The listing builds one solid part. Answer for the finished solid, in the listing's coordinates (mm). A direction names the side the tool comes from. Coordinates: 2 decimals unless noted, no trailing zeros. Loops run counter-clockwise (first coordinate to the right, second up) from the corner with the lowest first, then second, coordinate; pieces in that order, holes last. Notation, with made-up numbers: M 44,-39 L 83,-39 A19 ccw 83,-26 Z; hole C 56.5,59 d8. An arc over 180 degrees is marked long. Return JSON: item names as keys, results as strings. Group by question number.
1. Section C-C (z = 29) is taken. Write down the section's boundary in (x, y).
2. Section D-D (y = 0) is taken. Write down the section's boundary in (x, z).
3. Given P1, Ø6, axis at x = -2.5, y = 39.5, coming from the +Z side, flat-ended and moving along its own axis, determine where the tip first touches the part or whether it passes through.
4. Section B-B (x = 31) is taken. Write down the section's boundary in (y, z), then the cut area to 3 significant figures.
5. Which of the six approach directions +Z, -Z, +X, -X, +Y, -Y give full straight-line access (tool end or side, diameter ignored) to faces 4 (the face through (-51, 1, 76.2)), 5 (the face through (-50.062, -1, 38)), 6 (the face through (26.223, -39, 63))?
6. Straight lines are drawn through the part: L1, parallel to X at y = 3, z = 32; L2, parallel to Y at x = 40, z = 63.5; L3, parallel to Z at x = -52.5, y = 0. For each, find the intervals that lie inside material, in ascending order. Write a range as from..to.
7. Section A-A (y = 24.5) is taken. Write down the section's boundary in (x, z).
8. The mould has two halves that part along Y. Classify faces 1 (the face through (26.223, 39, 63)), 2 (the face through (52.782, -1.485, 63.907)), 3 (the face through (-1, 41.569, 29)): pulls with the +Y half, pulls with the -Y half, needs draft (parallel to the pull), parting line crosses it, or undercut.
```python
from build123d import *

# Parameters (mm, degrees)
F0_W     = 110.851846
F0_H     = 83.138884
F0_W_2   = 100.124248
F0_H_2   = 71.815304
F1_DEPTH = 76.2
F2_W     = 52.446034
F2_H     = 26.882852
F3_DEPTH = 103.124
F4_R     = 11.409512
F5_DEPTH = 113.538


with BuildPart() as f1:
    # F0 (on Top) → F1 (new body)
    with BuildSketch(Plane.XY):
        Rectangle(F0_W, F0_H)
        Rectangle(F0_W_2, F0_H_2, mode=Mode.SUBTRACT)
    extrude(amount=F1_DEPTH)

    # F2 (on face) → F3 (cut)
    with BuildSketch(Plane.XZ.offset(41.569442)):
        with Locations((0, 62.758574)):
            Rectangle(F2_W, F2_H)
    extrude(amount=-F3_DEPTH, mode=Mode.SUBTRACT)

    # F4 (on face) → F5 (cut)
    with BuildSketch(Plane.YZ.offset(55.425923)):
        with Locations((0, 52.595027)):
            Circle(F4_R)
    extrude(amount=-F5_DEPTH, mode=Mode.SUBTRACT)


solid = f1.part
```
Worked out:
{
 "1": {"outline": "M -55.43,-41.57 L 55.43,-41.57 L 55.43,41.57 L -55.43,41.57 Z; hole M -50.06,-35.91 L 50.06,-35.91 L 50.06,35.91 L -50.06,35.91 Z"},
 "2": {"outline": "M -55.43,0 L -50.06,0 L -50.06,41.19 L -55.43,41.19 Z; M -55.43,64 L -50.06,64 L -50.06,76.2 L -55.43,76.2 Z; M 50.06,0 L 55.43,0 L 55.43,41.19 L 50.06,41.19 Z; M 50.06,64 L 55.43,64 L 55.43,76.2 L 50.06,76.2 Z"},
 "3": {"P1": "z = 49.32"},
 "4": {"outline": "M -41.57,0 L -35.91,0 L -35.91,76.2 L -41.57,76.2 Z; M 35.91,0 L 41.57,0 L 41.57,76.2 L 35.91,76.2 Z", "area": "863 mm^2"},
 "5": {"face 4": "+Z, +X, -X, +Y, -Y", "face 5": "+Z, -Z", "face 6": "+Z, +Y, -Y"},
 "6": {"L1": "-55.43..-50.06, 50.06..55.43", "L2": "-41.57..-35.91, 35.91..41.57", "L3": "0..41.19, 64..76.2"},
 "7": {"outline": "M -55.43,0 L -50.06,0 L -50.06,76.2 L -55.43,76.2 Z; M 50.06,0 L 55.43,0 L 55.43,76.2 L 50.06,76.2 Z"},
 "8": {"face 1": "needs draft", "face 2": "undercut", "face 3": "pulls with the +Y half"}
}
